Verification items for this drawing (mm, ordinates from the low corner). A direction names the side the tool comes from. Give positions to 0.01 mm unless a question says otherwise; leave off trailing zeros. Loops run counter-clockwise (first coordinate to the right, second up) from the corner with the lowest first, then second, coordinate; pieces in that order, holes last. Notation, with made-up numbers: M 48,24 L 75,24 A28 ccw 75,62 Z; hole C 25.25,21 d7. An arc over 180 degrees is marked long. Write each question's results on one line, items separated by ' | '. Start each with the question number.
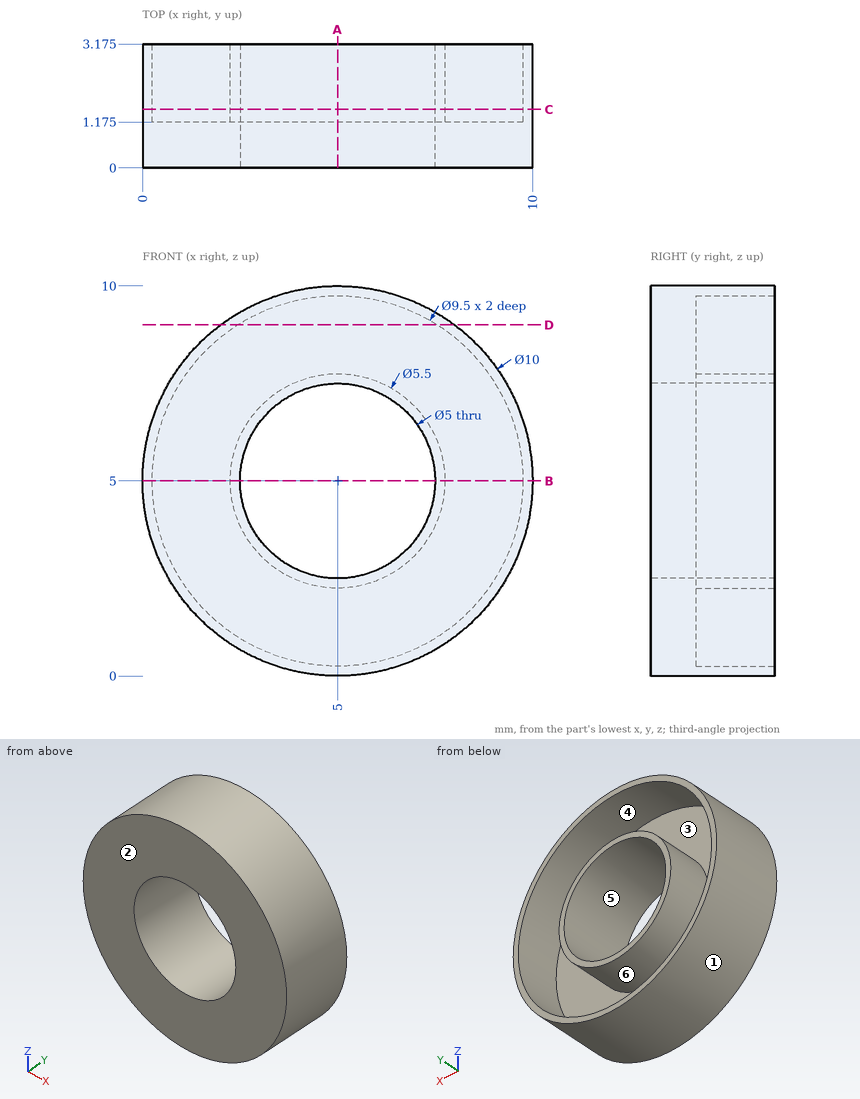
1. Set-up check for the marked faces 5 and 6: record each of +Z, -Z, +X, -X, +Y, -Y from which the full face is reachable in a straight line by a thin tool's end or side.
2. Section check A-A, the plane x = 5. Record the boundary of the cut face in (y, z) (3 decimals).
3. Section check D-D, the plane z = 9. Record the boundary of the cut face in (x, y) (3 decimals).
4. Release check for a two-part mould opening along Z. For the marked faces 1, 2, 3 and 4 record: released by +Z, released by -Z, zero draft, split by the parting line, or undercut.
5. Section check C-C, the plane y = 1.5. Record the boundary of the cut face in (x, z), plus the area to 3 significant figures.
6. Depth check by flat-ended pin: pin 1 Ø4 at (x, z) = (5, 5) entering from -Y. Enter the tip coordinate at first touch or a pass-through.
7. Thickness scan on probe 1 along X at (y, z) = (2.1, 5); probe 2 along X at (y, z) = (2.05, 4). Record the ranges inside material, lowest first.
8. Section check B-B, the plane z = 5. Record the boundary of the cut face in (x, y) (3 decimals), plus the area to 4 significant figures.
Filled sheet:
1) face 5: +Y, -Y | face 6: +Y
2) outline: M 0,0 L 3.175,0 L 3.175,0.25 L 1.175,0.25 L 1.175,2.25 L 3.175,2.25 L 3.175,2.5 L 0,2.5 Z; M 0,7.5 L 3.175,7.5 L 3.175,7.75 L 1.175,7.75 L 1.175,9.75 L 3.175,9.75 L 3.175,10 L 0,10 Z
3) outline: M 2,0 L 8,0 L 8,3.175 L 7.562,3.175 L 7.562,1.175 L 2.438,1.175 L 2.438,3.175 L 2,3.175 Z
4) face 1: split by the parting line | face 2: zero draft | face 3: undercut | face 4: undercut
5) outline: C 5,5 d10; C 5,5 d5.5; hole C 5,5 d9.5; hole C 5,5 d5 | area: 11.8 mm2
6) pin 1: through
7) probe 1: 0 to 0.25, 2.25 to 2.5, 7.5 to 7.75, 9.75 to 10 | probe 2: 0.1 to 0.36, 2.44 to 2.71, 7.29 to 7.56, 9.64 to 9.9
8) outline: M 0,0 L 2.5,0 L 2.5,3.175 L 2.25,3.175 L 2.25,1.175 L 0.25,1.175 L 0.25,3.175 L 0,3.175 Z; M 7.5,0 L 10,0 L 10,3.175 L 9.75,3.175 L 9.75,1.175 L 7.75,1.175 L 7.75,3.175 L 7.5,3.175 Z | area: 7.875 mm2
